```python
from build123d import *

# Parameters (mm, degrees)
SKETCH_1_R          = 20
SKETCH_1_R_2        = 15
EXTRUDE_1_DEPTH     = 3
SKETCH_2_R          = 2.5
CUT_EXTRUDE_1_DEPTH = 92.262525064
SKETCH_3_R          = 5
CUT_EXTRUDE_2_DEPTH = 10
SKETCH_4_R          = 5
SKETCH_4_R_2        = 4.25
EXTRUDE_2_DEPTH     = 3


with BuildPart() as part:
    # 草图1 → 凸台-拉伸1 (new body)
    with BuildSketch(Plane(origin=(0, 0, 0), x_dir=(1, 0, 0), z_dir=(0, 1, 0))):
        Circle(SKETCH_1_R)
        with BuildLine():
            ThreePointArc((20, 0), (8.309115435, -18.192267607), (-13.095860068, -15.116165158))
            Line((-13.095860068, -15.116165158), (39.675579632, -60.834598551))
            ThreePointArc((39.675579632, -60.834598551), (38.890872965, -38.890872965), (60.834598551, -39.675579632))
            Line((60.834598551, -39.675579632), (15.116165158, 13.095860068))
            ThreePointArc((15.116165158, 13.095860068), (18.73930766, 6.98844392), (20, 0))
        make_face()
        with Locations((49.497474683, -49.497474683)):
            Circle(SKETCH_1_R_2)
    extrude(amount=EXTRUDE_1_DEPTH)

    # 草图2 → 切除-拉伸1 (cut, through all)
    with BuildSketch(Plane(origin=(0, 3, 0), x_dir=(1, 0, 0), z_dir=(0, 1, 0))):
        with Locations(Location((0, 0, 0), (0, 0, 270))):
            Circle(SKETCH_2_R)
    extrude(amount=-CUT_EXTRUDE_1_DEPTH, mode=Mode.SUBTRACT)

    # 草图3 → 切除-拉伸2 (cut)
    with BuildSketch(Plane(origin=(0, 3, 0), x_dir=(1, 0, 0), z_dir=(0, 1, 0))):
        with Locations(Location((0, 0, 0), (0, 0, 270))):
            Circle(SKETCH_3_R)
    extrude(amount=-CUT_EXTRUDE_2_DEPTH, mode=Mode.SUBTRACT)

    # 草图4 → 凸台-拉伸2 (add)
    with BuildSketch(Plane(origin=(0, 3, 0), x_dir=(1, 0, 0), z_dir=(0, 1, 0))):
        Circle(SKETCH_4_R)
        with Locations(Location((0, 0, 0), (0, 0, 270))):
            Circle(SKETCH_4_R_2, mode=Mode.SUBTRACT)
    extrude(amount=-EXTRUDE_2_DEPTH)


solid = part.part
```
Geometry check sheet. Reference: the model listing, model coordinates, mm. Give positions to 0.01 mm unless a question says otherwise; leave off trailing zeros. Order: outer loops, then holes, each group sorted by start corner. A loop starts at its lowest first (then second) coordinate and runs counter-clockwise, first axis right, second up.
1. Section check A-A, the plane z = 0. Enter the section's corners in (x, y).
2. Section check C-C, the plane y = 2.2. Enter the section's corners in (x, z).
3. Section check D-D, the plane x = 48.5. Enter the section's corners in (y, z), and give its area (3 significant figures).
4. Thickness scan on L1, parallel to X at y = 1.8, z = 0; L2, parallel to Z at x = -1.5, y = 2.45; L3, parallel to Z at x = -3.5, y = 0.85. Record the ranges inside material, lowest first.
5. Gauge pin test, flat end, axial feed: pin 1 Ø1.5 at (x, y) = (37.5, 2) entering from -Z. Record the tip position at first contact, or that the pin passes through.
6. Release check for a two-part mould opening along Z. For faces 1 (the face through (4.214, 1.521, -0.553)), 2 (the face through (38.295, 1.479, 13.659)), 3 (the face through (-13.813, 1.479, -14.464)) record: pulls with the +Z half, pulls with the -Z half, needs draft (parallel to the pull), parting line crosses it, or undercut.
7. Section check B-B, the plane x = 0. Enter the section's corners in (y, z), and give its area (3 significant figures).
Values follow:
1. outline: (-20, 0) - (-4.25, 0) - (-4.25, 3) - (-20, 3) - close; (4.25, 0) - (26.46, 0) - (26.46, 3) - (4.25, 3) - close
2. outline: (-13.1, 15.12) arc R20 ccw (long way) to (15.12, -13.1) - (60.83, 39.68) arc R15 ccw to (39.68, 60.83) - close; hole circle Ø8.5 at (0, 0)
3. outline: (0, 25.44) - (3, 25.44) - (3, 64.46) - (0, 64.46) - close
3. area: 117 mm2
4. L1: x = -20 to -4.25, 4.25 to 26.46
4. L2: z = -19.94 to -3.98, 3.98 to 25.16
4. L3: z = -19.69 to -2.41, 2.41 to 23.43
5. pin 1: stops at z = 11.88
6. face 1: undercut
6. face 2: pulls with the -Z half
6. face 3: parting line crosses it
7. outline: (0, -20) - (3, -20) - (3, -4.25) - (0, -4.25) - close; (0, 4.25) - (3, 4.25) - (3, 26.46) - (0, 26.46) - close
7. area: 114 mm2
